from build123d import *

# Parameters (mm, degrees)
SKIZZE1_R                       = 10
AUFSATZ_LINEAR_AUSTRAGEN1_DEPTH = 12
SKIZZE2_R                       = 3.9
AUFSATZ_LINEAR_AUSTRAGEN2_DEPTH = 4
SKIZZE3_R                       = 2.2
SCHNITT_LINEAR_AUSTRAGEN1_DEPTH = 8
SCHNITT_LINEAR_AUSTRAGEN2_REACH = 22
SKIZZE4_R                       = 1.25
SKIZZE5_R                       = 1.2
SCHNITT_LINEAR_AUSTRAGEN3_DEPTH = 9


with BuildPart() as part:
    # Skizze1 → Aufsatz-Linear austragen1 (new body)
    with BuildSketch(Plane(origin=(0, 0, 0), x_dir=(1, 0, 0), z_dir=(0, 1, 0))):
        Circle(SKIZZE1_R)
    extrude(amount=AUFSATZ_LINEAR_AUSTRAGEN1_DEPTH)

    # Skizze2 → Aufsatz-Linear austragen2 (add)
    with BuildSketch(Plane(origin=(0, 12, 0), x_dir=(1, 0, 0), z_dir=(0, 1, 0))):
        Circle(SKIZZE2_R)
    extrude(amount=AUFSATZ_LINEAR_AUSTRAGEN2_DEPTH)

    # Skizze3 → Schnitt-Linear austragen1 (cut)
    with BuildSketch(Plane.XZ):
        Circle(SKIZZE3_R)
    extrude(amount=-SCHNITT_LINEAR_AUSTRAGEN1_DEPTH, mode=Mode.SUBTRACT)

    # Skizze4 → Schnitt-Linear austragen2 (cut, up to next)
    with BuildSketch(Plane.XY.offset(10), mode=Mode.PRIVATE) as schnitt_linear_austragen2_sk1:
        with Locations((0, 3.5)):
            Circle(SKIZZE4_R)
    schnitt_linear_austragen2_tool1 = extrude(schnitt_linear_austragen2_sk1.sketch, amount=-SCHNITT_LINEAR_AUSTRAGEN2_REACH, mode=Mode.PRIVATE) & part.part
    add(schnitt_linear_austragen2_tool1.solids().sort_by_distance((0, 3.5, 10))[0], mode=Mode.SUBTRACT)

    # Skizze5 → Schnitt-Linear austragen3 (cut)
    with BuildSketch(Plane(origin=(0, 12, 0), x_dir=(1, 0, 0), z_dir=(0, 1, 0))):
        with Locations((-5.25, 5.25)):
            Circle(SKIZZE5_R)
        with Locations((5.25, 5.25)):
            Circle(SKIZZE5_R)
        with Locations((5.25, -5.25)):
            Circle(SKIZZE5_R)
        with Locations((-5.25, -5.25)):
            Circle(SKIZZE5_R)
    extrude(amount=-SCHNITT_LINEAR_AUSTRAGEN3_DEPTH, mode=Mode.SUBTRACT)


solid = part.part
The listing builds one solid part. Answer for the finished solid, in the listing's coordinates (mm). A direction names the side the tool comes from. Round coordinates to 2 decimals unless told otherwise and drop trailing zeros. Order: outer loops, then holes, each group sorted by start corner. A loop starts at its lowest first (then second) coordinate and runs counter-clockwise, first axis right, second up. Notation, with made-up numbers: (9.25, 0.25) -> (25.25, 0.25) arc R21 ccw to (25.25, 19.25) -> close; hole circle Ø4 at (-30, -2). An arc over 180 degrees is marked (long way). Write each question's results on one line, items separated by ' | '. Start each with the question number.
Q1. Find section A-A (x = 0). Determine the outline of the cut face in (y, z), then the cut area to 4 significant figures.
Q2. The mould has two halves that part along Z. Classify faces 5 (the cylindrical face through (-2.87, 13.97, -2.64)), 6 (the flat face through (5, 3, 5)), 7 (the cylindrical face through (-6.45, 7.56, -5.3)), 8 (the flat face through (0, 16, 0)): pulls with the +Z half, pulls with the -Z half, needs draft (parallel to the pull), parting line crosses it, or undercut.
Q3. Straight lines are drawn through the part: probe 1 along X at (y, z) = (3.5, 5); probe 2 along Z at (x, y) = (5.25, 9.5); probe 3 along Y at (x, z) = (0, 6.75). For each, find the intervals that lie inside material, in ascending order. Write a range as from..to.
Q4. Find section D-D (y = 10.5). Determine the outline of the cut face in (x, z), then the cut area to 3 significant figures.
Q5. Each of these flat-tipped pins is pushed along its axis until it touches: pin 1 (1 mm diameter, centred on y = 12, z = 5, fed in from +X); pin 2 (1.2 mm diameter, centred on x = 5, z = -5.5, fed in from +Y); pin 3 (3 mm diameter, centred on x = 6, y = 12, fed in from +Z); pin 4 (5 mm diameter, centred on y = 2, z = 1, fed in from +X). Where does it stop, or does it pass through?
Q6. Find section B-B (z = 0). Determine the outline of the cut face in (x, y), then the cut area to 3 significant figures.
Q7. Find section C-C (y = 6.25). Determine the outline of the cut face in (x, z), then the cut area to 3 significant figures.
Q8. Which of the six approach directions +Z, -Z, +X, -X, +Y, -Y give full straight-line access (tool end or side, diameter ignored) to faces 1 (the cylindrical face through (-0.27, 2.28, 5.96)), 2 (the flat face through (-0.1, 0, -2.4)), 3 (the cylindrical face through (1.02, 3.94, -1.95)), 4 (the flat face through (-5, 3, 5))?
Worked answers:
1) outline: (0, -10) -> (12, -10) -> (12, -3.9) -> (16, -3.9) -> (16, 3.9) -> (12, 3.9) -> (12, 10) -> (4.75, 10) -> (4.75, 2.2) -> (8, 2.2) -> (8, -2.2) -> (0, -2.2) -> close; (0, 2.2) -> (2.25, 2.2) -> (2.25, 10) -> (0, 10) -> close | area: 216.5 mm2
2) face 5: parting line crosses it | face 6: undercut | face 7: undercut | face 8: needs draft
3) probe 1: x = -8.66..-6.42, -4.08..-1.25, 1.25..4.08, 6.42..8.66 | probe 2: z = -8.51..-6.45, -4.05..4.05, 6.45..8.51 | probe 3: y = 0..2.25, 4.75..12
4) outline: circle Ø20 at (0, 0); hole circle Ø2.4 at (-5.25, -5.25); hole circle Ø2.4 at (-5.25, 5.25); hole circle Ø2.4 at (5.25, -5.25); hole circle Ø2.4 at (5.25, 5.25) | area: 296 mm2
5) pin 1: stops at x = 8.93 | pin 2: stops at y = 3 | pin 3: stops at z = 8.93 | pin 4: stops at x = 10
6) outline: (-10, 0) -> (-2.2, 0) -> (-2.2, 8) -> (2.2, 8) -> (2.2, 0) -> (10, 0) -> (10, 12) -> (3.9, 12) -> (3.9, 16) -> (-3.9, 16) -> (-3.9, 12) -> (-10, 12) -> close | area: 236 mm2
7) outline: circle Ø20 at (0, 0); hole circle Ø2.4 at (-5.25, -5.25); hole circle Ø2.4 at (-5.25, 5.25); hole circle Ø4.4 at (0, 0); hole circle Ø2.4 at (5.25, -5.25); hole circle Ø2.4 at (5.25, 5.25) | area: 281 mm2
8) face 1: +Z | face 2: +Z, -Z, +X, -X, -Y | face 3: -Y | face 4: +Y
